Verification items for the finished model (mm, model axes). A direction names the side the tool comes from. Round coordinates to 2 decimals unless told otherwise and drop trailing zeros. Write each loop counter-clockwise with the first axis right and the second up, starting at its lowest first coordinate (ties: lowest second). Pieces come first, ordered by that corner, then holes. Notation, with made-up numbers: M -2,24 L 45,24 A21 cw 45,41 Z; hole C 67.25,76.25 d9. An arc over 180 degrees is marked long. One line per question, with ' | ' between items. Start each with the question number.
Q1. Cross-section at A-A (x = -29.35). Record the boundary of the cut face in (y, z).
Q2. Gauge pin test, flat end, axial feed: pin 1 (1.5 mm diameter, centred on x = -20.5, z = 0, fed in from -Y). Record the tip position at first contact, or that the pin passes through.
Q3. Thickness scan on line 1 along X through (y, z) = (15, 0); line 2 along X through (y, z) = (2.75, 0); line 3 along Z through (x, y) = (-29.35, 15.5). Record the ranges inside material, lowest first. Write a range as from..to.
Q4. Tool access check on faces 4 (the face through (-21.265, 4.93, 0.806)), 5 (the face through (-27.886, 13.14, 0.325)), 6 (the face through (-1, 18.07, 0)). Record the directions out of +Z, -Z, +X, -X, +Y, -Y that give a thin tool (end or side, any length) a straight path to the whole face; none if there is none.
Q5. Release check for a two-part mould opening along X. For faces 1 (the face through (-20, 10, 0)), 2 (the face through (-38.3, 9, 0)), 3 (the face through (-1, 0, 0)) record: released by +X, released by -X, zero draft, split by the parting line, or undercut.
Q6. Cross-section at B-B (z = 0). Record the boundary of the cut face in (x, y), then the cut area to 3 significant figures.
from build123d import *

# Parameters (mm, degrees)
SKETCH_1_W          = 76.6
SKETCH_1_H          = 42.4
EXTRUDE_1_DEPTH     = 18.07
SKETCH_2_R          = 1.5
CUT_EXTRUDE_1_DEPTH = 10
SKETCH_3_R          = 1.5
CUT_EXTRUDE_2_DEPTH = 10


with BuildPart() as part:
    # Эскиз1 → Бобышка-Вытянуть1 (new body)
    with BuildSketch(Plane(origin=(0, 0, 0), x_dir=(1, 0, 0), z_dir=(0, 1, 0))):
        Rectangle(SKETCH_1_W, SKETCH_1_H)
    extrude(amount=EXTRUDE_1_DEPTH)

    # Эскиз2 → Вырез-Вытянуть1 (cut)
    with BuildSketch(Plane(origin=(0, 18.07, 0), x_dir=(1, 0, 0), z_dir=(0, 1, 0))):
        with Locations(Location((29.35, 0, 0), (0, 0, 270))):
            Circle(SKETCH_2_R)
        with Locations(Location((-29.35, 0, 0), (0, 0, 90))):
            Circle(SKETCH_2_R)
    extrude(amount=-CUT_EXTRUDE_1_DEPTH, mode=Mode.SUBTRACT)

    # Эскиз3 → Вырез-Вытянуть2 (cut)
    with BuildSketch(Plane.XZ):
        with Locations(Location((20, 0, 0), (0, 0, 270))):
            Circle(SKETCH_3_R)
        with Locations(Location((-20, 0, 0), (0, 0, 90))):
            Circle(SKETCH_3_R)
    extrude(amount=-CUT_EXTRUDE_2_DEPTH, mode=Mode.SUBTRACT)


solid = part.part
Determined:
1) outline: M 0,-21.2 L 18.07,-21.2 L 18.07,-1.5 L 8.07,-1.5 L 8.07,1.5 L 18.07,1.5 L 18.07,21.2 L 0,21.2 Z
2) pin 1: stops at y = 10
3) line 1: x = -38.3..-30.85, -27.85..27.85, 30.85..38.3 | line 2: x = -38.3..-21.5, -18.5..18.5, 21.5..38.3 | line 3: z = -21.2..-1.5, 1.5..21.2
4) face 4: -Y | face 5: +Y | face 6: +Z, -Z, +X, -X, +Y
5) face 1: undercut | face 2: released by -X | face 3: zero draft
6) outline: M -38.3,0 L -21.5,0 L -21.5,10 L -18.5,10 L -18.5,0 L 18.5,0 L 18.5,10 L 21.5,10 L 21.5,0 L 38.3,0 L 38.3,18.07 L 30.85,18.07 L 30.85,8.07 L 27.85,8.07 L 27.85,18.07 L -27.85,18.07 L -27.85,8.07 L -30.85,8.07 L -30.85,18.07 L -38.3,18.07 Z | area: 1,260 mm²
